Geometry check sheet. Reference: the model listing, model coordinates, mm. A direction names the side the tool comes from. Coordinates: 2 decimals unless noted, no trailing zeros. Order: outer loops, then holes, each group sorted by start corner. A loop starts at its lowest first (then second) coordinate and runs counter-clockwise, first axis right, second up. Notation, with made-up numbers: (-14.5, 19) - (-7.5, 19) arc R22 cw to (-7.5, 32) - close; hole circle Ø1 at (37.25, 88.25). An arc over 180 degrees is marked (long way). Put each result on its own line as item: value.
Autodesk Inventor part; units mm, degrees
ref_plane "YZ Plane" through (0, 0, 0) normal (1, 0, 0) x (0, 1, 0)
ref_plane "XZ Plane" through (0, 0, 0) normal (0, 1, 0) x (-1, 0, 0)
ref_plane "XY Plane" through (0, 0, 0) normal (0, 0, 1) x (1, 0, 0)
sketch "Sketch1" plane through (0, 0, 0) normal (0, 0, 1) x (1, 0, 0)
  line L0 (-70, -10) -> (70, -10)
  line L1 (70, -10) -> (70, 10)
  line L2 (70, 10) -> (-70, 10)
  line L3 (-70, 10) -> (-70, -10)
  line L4 (-70, -10) -> (70, 10) construction
  line L5 (70, -10) -> (-70, 10) construction
  circle A0 centre (0, 0) radius 16
  line L6 (-73.4722, 0) -> (96.5278, 0) construction
  circle A1 centre (-60, 0) radius 2.75
  line L7 (0, 0) -> (0, 31) construction
  circle A2 centre (60, 0) radius 2.75
  circle A3 centre (0, 0) radius 1.5
  circle A4 centre (-6.9148, 6.9148) radius 1.7526
  line L8 (0, 0) -> (-14.5685, 14.5685) construction
  circle A5 centre (-6.9148, -6.9148) radius 1.7526
  circle A6 centre (6.9148, -6.9148) radius 1.7526
  circle A7 centre (6.9148, 6.9148) radius 1.7526
  point P0 (0, 0)
  dimension "d0" = 140
  dimension "d1" = 20
  dimension "d4" = 32
  dimension "d5" = 5.5
  dimension "d6" = 10
  dimension "d10" = 3
  dimension "d11" = 3.5052
  dimension "d12" = 45
  dimension "d13" = 6.9148
  dimension "d16" = 360
extrude "Extrusion1" add sketch "Sketch1" along normal blind 5 contours L3 L2 A0 L0 | A0 L2 L0 | L0 A0 | A0 L2 L1 L0 | A0 L2 | A1 | A2 | A3 | A4 | A5 | A6 | A7
extrude "Extrusion2" cut sketch "Sketch1" along normal through all contours A1 | A2 | A3 | A4 | A5 | A6 | A7
fillet "Fillet1" radius 5 4 edges at (70, -10, 2.5) (70, 10, 2.5) (-70, -10, 2.5) (-70, 10, 2.5)
equation "\"BendRadius\" = Thickness"
equation "\"BendReliefWidth\" = Thickness"
equation "\"BendReliefDepth\" = 0.5 * Thickness"
equation "\"CornerReliefSize\" = 4 * Thickness"
equation "\"MinimumRemnant\" = 2 * Thickness"
equation "\"TransitionRadius\" = BendRadius"
equation "\"JacobiRadiusSize\" = Thickness"
equation "\"GapSize\" = Thickness"
properties part number "rudder_horn"
Q1. Draft check along X on faces 5 (the flat face through (-1, 4, 0)), 6 (the cylindrical face through (0, -16, 2)), 7 (the cylindrical face through (6.687, -8.652, 2.465)). Enter one of: pulls with the +X half, pulls with the -X half, needs draft (parallel to the pull), parting line crosses it, or undercut.
Answer block:
face 5: needs draft
face 6: parting line crosses it
face 7: undercut
Q2. Access from +Z, -Z, +X, -X, +Y, -Y to the whole of each face (thin tool, end or side, straight path). Record for faces 1 (the flat face through (38, -10, 2)), 2 (the flat face through (-38, 10, 2)), 3 (the flat face through (39, 10, 2)), 4 (the flat face through (-39, -10, 2)).
Answer block:
face 1: +Z, -Z, +X, -Y
face 2: +Z, -Z, -X, +Y
face 3: +Z, -Z, +X, +Y
face 4: +Z, -Z, -X, -Y
Q3. Depth check by flat-ended pin: pin 1 Ø2 at (x, y) = (-6.91, -6.91) entering from -Z; pin 2 Ø1 at (y, z) = (-12.5, 4.5) entering from +X; pin 3 Ø1 at (x, z) = (21, 1) entering from -Y; pin 4 Ø2.5 at (x, z) = (-44.5, 3) entering from +Y. Enter the tip coordinate at first touch or a pass-through.
Answer block:
pin 1: passes through
pin 2: stops at x = 10.58
pin 3: stops at y = -10
pin 4: stops at y = 10
Q4. Section check B-B on y = 0. Record the boundary of the cut face in (x, z).
Answer block:
outline: (-70, 0) - (-62.75, 0) - (-62.75, 5) - (-70, 5) - close; (-57.25, 0) - (-1.5, 0) - (-1.5, 5) - (-57.25, 5) - close; (1.5, 0) - (57.25, 0) - (57.25, 5) - (1.5, 5) - close; (62.75, 0) - (70, 0) - (70, 5) - (62.75, 5) - close
Q5. Section check A-A on x = -60. Record the boundary of the cut face in (y, z).
Answer block:
outline: (-10, 0) - (-2.75, 0) - (-2.75, 5) - (-10, 5) - close; (2.75, 0) - (10, 0) - (10, 5) - (2.75, 5) - close
Q6. Section check C-C on x = 0. Record the boundary of the cut face in (y, z), then the cut area to 3 significant figures.
Answer block:
outline: (-16, 0) - (-1.5, 0) - (-1.5, 5) - (-16, 5) - close; (1.5, 0) - (16, 0) - (16, 5) - (1.5, 5) - close
area: 145 mm^2
Q7. Thickness scan on L1, parallel to X at y = 0, z = 1.3; L2, parallel to Y at x = -60, z = 3.65; L3, parallel to Y at x = 6, z = 3.7. Record the ranges inside material, lowest first. Write a range as [from, to].
Answer block:
L1: x = [-70, -62.75], [-57.25, -1.5], [1.5, 57.25], [62.75, 70]
L2: y = [-10, -2.75], [2.75, 10]
L3: y = [-14.83, -8.41], [-5.42, 5.42], [8.41, 14.83]
Q8. Section check D-D on z = 3.85. Record the boundary of the cut face in (x, y), then the cut area to 3 significant figures.
Answer block:
outline: (-70, -5) arc R5 ccw to (-65, -10) - (-12.49, -10) arc R16 ccw to (12.49, -10) - (65, -10) arc R5 ccw to (70, -5) - (70, 5) arc R5 ccw to (65, 10) - (12.49, 10) arc R16 ccw to (-12.49, 10) - (-65, 10) arc R5 ccw to (-70, 5) - close; hole circle Ø5.5 at (-60, 0); hole circle Ø3.51 at (-6.91, -6.91); hole circle Ø3.51 at (-6.91, 6.91); hole circle Ø3 at (0, 0); hole circle Ø3.51 at (6.91, -6.91); hole circle Ø3.51 at (6.91, 6.91); hole circle Ø5.5 at (60, 0)
area: 2,890 mm^2
